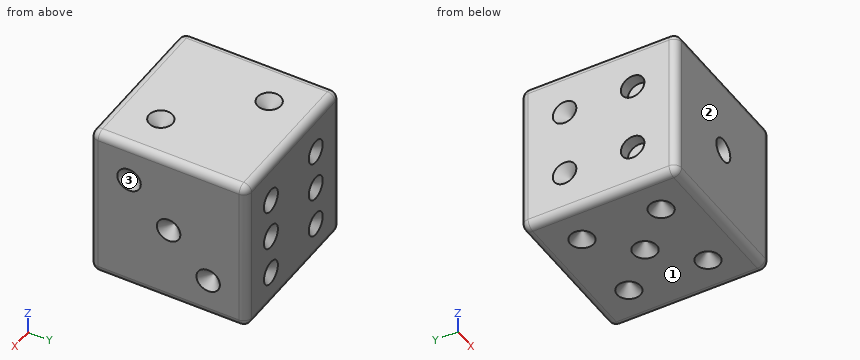
from build123d import *

# Parameters (mm, degrees)
F0_W      = 20
F0_H      = 20
F1_DEPTH  = 20
F2_R      = 1.5
F3_DEPTH  = 1.5
F4_R      = 1.5
F5_DEPTH  = 1.5
F6_R      = 1
F7_SIZE   = 1.49999
F8_R      = 1.5
F9_DEPTH  = 1.5
F10_SIZE  = 1.49999
F11_R     = 1.5
F12_DEPTH = 1.5
F13_SIZE  = 1.49999
F14_R     = 1.5
F15_DEPTH = 1.5
F16_SIZE  = 1.49999
F17_R     = 1.5
F18_DEPTH = 1.5
F19_SIZE  = 1.49999


# Not quite as in the source:
# - a fillet or chamfer is up to 0.001 mm smaller than in the source, because OpenCascade refuses the exact size


with BuildPart() as f1:
    # F0 (on Top) → F1 (new body)
    with BuildSketch(Plane.XY):
        with Locations((10, 10)):
            Rectangle(F0_W, F0_H)
    extrude(amount=F1_DEPTH)

    # F2 (on face) → F3 (cut)
    with BuildSketch(Plane.XZ):
        with Locations((10, 10)):
            Circle(F2_R)
    extrude(amount=-F3_DEPTH, mode=Mode.SUBTRACT)

    # F4 (on face) → F5 (cut)
    with BuildSketch(Plane.XY.offset(20)):
        with Locations((14.3431457505, 5.6568542495)):
            Circle(F4_R)
        with Locations((5.6568542495, 14.3431457505)):
            Circle(F4_R)
    extrude(amount=-F5_DEPTH, mode=Mode.SUBTRACT)

    # F6
    f6_edges = [f1.edges().sort_by_distance(p)[0] for p in [
        (0, 10, 20),
        (10, 20, 20),
        (20, 10, 20),
        (20, 10, 0),
        (10, 0, 20),
        (10, 0, 0),
        (0, 0, 10),
        (20, 0, 10),
        (20, 20, 10),
        (10, 20, 0),
        (0, 10, 0),
        (0, 20, 10),
    ]]
    fillet(f6_edges, radius=F6_R)

    # F7 (size 1.5 in the source; OpenCascade refuses exactly that, so slightly less here)
    f7_edges = [f1.edges().sort_by_distance(p)[0] for p in [
        (12.843146, 5.656854, 18.5),
        (4.156854, 14.343146, 18.5),
        (8.5, 1.5, 10),
    ]]
    chamfer(f7_edges, length=F7_SIZE)

    # F8 (on face) → F9 (cut)
    with BuildSketch(Plane.YZ.offset(20)):
        with Locations((15.0502525317, 4.9497474683)):
            Circle(F8_R)
        with Locations((4.9497474683, 15.0502525317)):
            Circle(F8_R)
        with Locations((10, 10)):
            Circle(F8_R)
    extrude(amount=-F9_DEPTH, mode=Mode.SUBTRACT)

    # F10 (size 1.5 in the source; OpenCascade refuses exactly that, so slightly less here)
    f10_edges = [f1.edges().sort_by_distance(p)[0] for p in [
        (18.5, 3.449747, 15.050253),
        (18.5, 8.5, 10),
        (18.5, 13.550253, 4.949747),
    ]]
    chamfer(f10_edges, length=F10_SIZE)

    # F11 (on face) → F12 (cut)
    with BuildSketch(Plane(origin=(0, 0, 0), x_dir=(0, -1, 0), z_dir=(-1, 0, 0))):
        with Locations((-14.3431457505, 14.3431457505)):
            Circle(F11_R)
        with Locations((-14.3431457505, 5.6568542495)):
            Circle(F11_R)
        with Locations((-5.6568542495, 14.3431457505)):
            Circle(F11_R)
        with Locations((-5.6568542495, 5.6568542495)):
            Circle(F11_R)
    extrude(amount=-F12_DEPTH, mode=Mode.SUBTRACT)

    # F13 (size 1.5 in the source; OpenCascade refuses exactly that, so slightly less here)
    f13_edges = [f1.edges().sort_by_distance(p)[0] for p in [
        (1.5, 15.843146, 14.343146),
        (1.5, 15.843146, 5.656854),
    ]]
    chamfer(f13_edges, length=F13_SIZE)

    # F14 (on face) → F15 (cut)
    with BuildSketch(Plane(origin=(0, 0, 0), x_dir=(1, 0, 0), z_dir=(0, 0, -1))):
        with Locations((4.9497474683, -15.0502525317)):
            Circle(F14_R)
        with Locations((15.0502525317, -15.0502525317)):
            Circle(F14_R)
        with Locations((15.0502525317, -4.9497474683)):
            Circle(F14_R)
        with Locations((4.9497474683, -4.9497474683)):
            Circle(F14_R)
        with Locations((10, -10)):
            Circle(F14_R)
    extrude(amount=-F15_DEPTH, mode=Mode.SUBTRACT)

    # F16 (size 1.5 in the source; OpenCascade refuses exactly that, so slightly less here)
    f16_edges = [f1.edges().sort_by_distance(p)[0] for p in [
        (3.449747, 4.949747, 1.5),
        (13.550253, 4.949747, 1.5),
        (8.5, 10, 1.5),
        (3.449747, 15.050253, 1.5),
        (13.550253, 15.050253, 1.5),
    ]]
    chamfer(f16_edges, length=F16_SIZE)

    # F17 (on face) → F18 (cut)
    with BuildSketch(Plane(origin=(0, 20, 0), x_dir=(-1, 0, 0), z_dir=(0, 1, 0))):
        with Locations((-5.1666666667, 9.6666666667)):
            Circle(F17_R)
        with Locations((-5.1666666667, 14.8333333333)):
            Circle(F17_R)
        with Locations((-14.8333333333, 4.5)):
            Circle(F17_R)
        with Locations((-5.1666666667, 4.5)):
            Circle(F17_R)
        with Locations((-14.8333333333, 14.8333333333)):
            Circle(F17_R)
        with Locations((-14.8333333333, 9.6666666667)):
            Circle(F17_R)
    extrude(amount=-F18_DEPTH, mode=Mode.SUBTRACT)

    # F19 (size 1.5 in the source; OpenCascade refuses exactly that, so slightly less here)
    f19_edges = [f1.edges().sort_by_distance(p)[0] for p in [
        (16.333333, 18.5, 14.833333),
        (6.666667, 18.5, 14.833333),
        (6.666667, 18.5, 9.666667),
        (6.666667, 18.5, 4.5),
        (16.333333, 18.5, 4.5),
        (16.333333, 18.5, 9.666667),
    ]]
    chamfer(f19_edges, length=F19_SIZE)


solid = f1.part
Read the model definition and answer for the solid it produces. Units are mm, in the model's axes. Face numbers are marked on the shaded views. Give positions to 0.01 mm unless a question says otherwise; leave off trailing zeros. Answer as a JSON object with one key per item and string values. Group by question number.
1) The mould has two halves that part along Y. Classify the marked faces 1, 2 and 3: +Y half, -Y half, draft (parallel to the pull), parting line (faces both ways), or undercut.
2) Each of these flat-tipped pins is pushed along its axis until it touches: P1, Ø2.5, axis at x = 4.95, y = 4.95, coming from the -Z side; P2, Ø2.5, axis at y = 15.05, z = 4.95, coming from the +X side. Where does it stop, or does it pass through?
3) Consider L1, parallel to Y at x = 5, z = 1; L2, parallel to Z at x = 5.75, y = 19.25; L3, parallel to Y at x = 10.5, z = 10.25. Determine where each line is inside the solid, lowest interval first. Write a range as from..to.
Values follow:
{
 "1": {"face 1": "draft", "face 2": "-Y half", "face 3": "undercut"},
 "2": {"P1": "stops at z = 0.25", "P2": "stops at x = 19.75"},
 "3": {"L1": "y = 0..4.45, 5.45..14.55, 15.55..20", "L2": "z = 0.03..4.03, 4.97..9.2, 10.14..14.36, 15.3..19.97", "L3": "y = 0.94..20"}
}
